```python
from build123d import *

# Parameters (mm, degrees)
COVER_START          = 72
COVER_DEPTH          = 18
PUMP_START           = 72
SKETCH2_W            = 60
SKETCH2_H            = 70
PUMP_WEB_DEPTH       = 24
WATER_START          = 72
SKETCH3_R            = 45
WATER_PUMP_DEPTH     = 53
PUMP_START_2         = 125
SKETCH4_R            = 40
PUMP_PULLEY_DEPTH    = 12
SEAL_BORE_DEPTH      = 257.38624879
SEAL_BORE_DEPTH_BACK = 257.38624879
SKETCH5_R            = 30


with BuildPart() as part:
    # Sketch1 → Cover (new body)
    with BuildSketch(Plane.XY.offset(COVER_START)):
        with BuildLine():
            Line((-79.703306689, -70), (79.703306689, -70))
            ThreePointArc((79.703306689, -70), (83.674122068, -68.498069055), (85.656973949, -64.744208408))
            Line((85.656973949, -64.744208408), (94.412091509, 5.296732068))
            ThreePointArc((94.412091509, 5.296732068), (94.391822309, 9.918554009), (93.1952955, 14.382853785))
            Line((93.1952955, 14.382853785), (64.589736738, 83.853496495))
            ThreePointArc((64.589736738, 83.853496495), (57.96144488, 91.955984369), (47.945530965, 95))
            Line((47.945530965, 95), (-47.945530965, 95))
            ThreePointArc((-47.945530965, 95), (-57.96144488, 91.955984369), (-64.589736738, 83.853496495))
            Line((-64.589736738, 83.853496495), (-93.1952955, 14.382853785))
            ThreePointArc((-93.1952955, 14.382853785), (-94.391822309, 9.918554009), (-94.412091509, 5.296732068))
            Line((-94.412091509, 5.296732068), (-85.656973949, -64.744208408))
            ThreePointArc((-85.656973949, -64.744208408), (-83.674122068, -68.498069055), (-79.703306689, -70))
        make_face()
    extrude(amount=COVER_DEPTH)

    # Sketch2 → Pump Web (add)
    with BuildSketch(Plane.XY.offset(PUMP_START)):
        with Locations((0, 115)):
            Rectangle(SKETCH2_W, SKETCH2_H)
    extrude(amount=PUMP_WEB_DEPTH)

    # Sketch3 → Water Pump (add)
    with BuildSketch(Plane.XY.offset(WATER_START)):
        with Locations(Location((0, 150, 0), (0, 0, 228.189685104))):
            Circle(SKETCH3_R)
    extrude(amount=WATER_PUMP_DEPTH)

    # Sketch4 → Pump Pulley (add)
    with BuildSketch(Plane.XY.offset(PUMP_START_2)):
        with Locations((0, 150)):
            Circle(SKETCH4_R)
    extrude(amount=PUMP_PULLEY_DEPTH)

    # Sketch5 → Seal Bore (cut, two sides: drawn at the far end of the back side and taken through both)
    with BuildSketch(Plane.XY.offset(-SEAL_BORE_DEPTH_BACK)):
        Circle(SKETCH5_R)
    extrude(amount=SEAL_BORE_DEPTH + SEAL_BORE_DEPTH_BACK, mode=Mode.SUBTRACT)


solid = part.part
```
The model under review builds one solid part; all positions refer to its coordinate system, in mm. A direction names the side the tool comes from. Round coordinates to 2 decimals unless told otherwise and drop trailing zeros. Write each loop counter-clockwise with the first axis right and the second up, starting at its lowest first coordinate (ties: lowest second). Pieces come first, ordered by that corner, then holes.
(1) We need section B-B on y = 0. Give the boundary of the cut face in (x, z).
(2) Insertion check: pin 1 (3 mm diameter, centred on y = 119, z = 97.5, fed in from +X); pin 2 (2 mm diameter, centred on x = -4, y = -43, fed in from +Z); pin 3 (19 mm diameter, centred on y = 90, z = 89, fed in from +X). Each pin has a flat end and moves straight along its axis. Give the tip position at first contact, or say it passes through.
(3) We need section D-D on z = 132. Give the boundary of the cut face in (x, y), and give its area (3 significant figures).
(4) Wall thickness on L1, parallel to Y at x = 0, z = 77.75; L2, parallel to Z at x = -12, y = 76; L3, parallel to X at y = 0, z = 82: over which ranges is each line inside the solid? List them lowest first.
(5) We need section A-A on x = 0. Give the boundary of the cut face in (y, z).
(6) Mouldability with a two-part tool opening along Y and no side actions: class faces 4 (the flat face through (-90.1, -29.2, 80.9)), 5 (the flat face through (-1, 32, 90)), 6 (the flat face through (30, 102, 86)) as +Y half, -Y half, draft (parallel to the pull), parting line (faces both ways), or undercut.
(7) Machinability: for faces 1 (the flat face through (-39, 95, 81)), 2 (the flat face through (39, 95, 81)), 3 (the flat face through (0.4, 190.2, 125)), which of the approach directions +Z, -Z, +X, -X, +Y, -Y give a long, thin tool a straight path to every point of the face, cutting with its end or side? Answer none if there is none.
(8) We need section C-C on y = 150. Give the boundary of the cut face in (x, z).
Findings below:
1. outline: (-93.75, 72) - (-30, 72) - (-30, 90) - (-93.75, 90) - close; (30, 72) - (93.75, 72) - (93.75, 90) - (30, 90) - close
2. pin 1: stops at x = 33.98
2. pin 2: stops at z = 90
2. pin 3: stops at x = 65.97
3. outline: circle Ø80 at (0, 150)
3. area: 5,030 mm2
4. L1: y = -70 to -30, 30 to 195
4. L2: z = 72 to 90
4. L3: x = -93.75 to -30, 30 to 93.75
5. outline: (-70, 72) - (-30, 72) - (-30, 90) - (-70, 90) - close; (30, 72) - (195, 72) - (195, 125) - (190, 125) - (190, 137) - (110, 137) - (110, 125) - (105, 125) - (105, 96) - (80, 96) - (80, 90) - (30, 90) - close
6. face 4: -Y half
6. face 5: draft
6. face 6: undercut
7. face 1: +Z, -Z, -X
7. face 2: +Z, -Z, +X
7. face 3: +Z
8. outline: (-45, 72) - (45, 72) - (45, 125) - (40, 125) - (40, 137) - (-40, 137) - (-40, 125) - (-45, 125) - close
